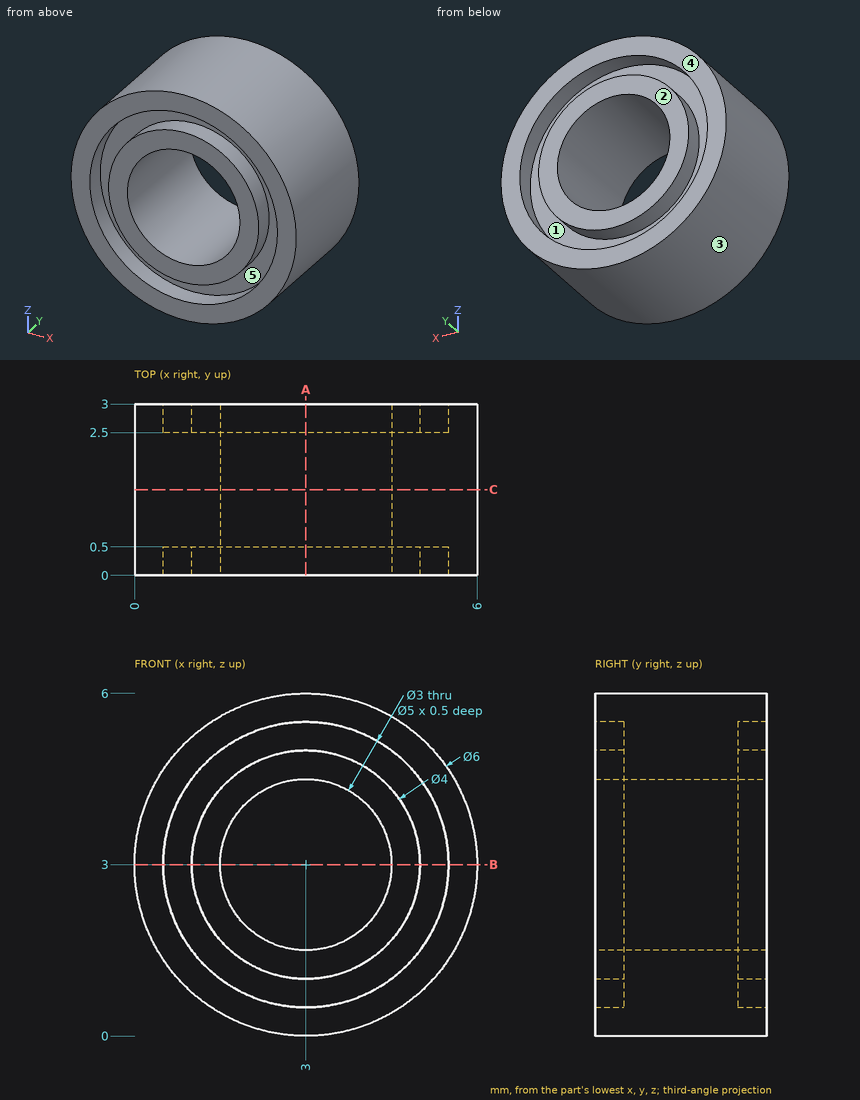
Geometry: see drawing. Coordinates: mm, zero at the bounding-box minimum. A direction names the side the tool comes from. Give positions to 0.01 mm unless a question says otherwise; leave off trailing zeros. Loops run counter-clockwise (first coordinate to the right, second up) from the corner with the lowest first, then second, coordinate; pieces in that order, holes last. Notation, with made-up numbers: (16.5, -34.75) -> (56.5, -34.75) arc R28 ccw to (56.5, -16.75) -> close; hole circle Ø8 at (10, 18.25). An arc over 180 degrees is marked (long way). Answer as a JSON object with one key per item and string values. Group by question number.
Item 1: Line query: probe 1 along X at (y, z) = (0.1, 3); probe 2 along Z at (x, y) = (1.45, 0.3); probe 3 along Z at (x, y) = (2.45, 0.2). Output: solid intervals per line, ascending.
Item 2: Pull-direction query (Z, two-part tool) for the marked faces 3, 4 and 5; classes: released by +Z, released by -Z, zero draft, split by the parting line, or undercut.
Item 3: Cut plane A-A, the plane x = 3. Return the cut outline in (y, z), and give its area (3 significant figures).
Item 4: Cut plane C-C, the plane y = 1.5. Return the cut outline in (x, z), and give its area (3 significant figures).
Item 5: Reachability of the marked faces 1 and 2 from +Z, -Z, +X, -X, +Y, -Y: full face, straight path, thin tool, end or side. Return the list, or none.
Item 6: Cut plane B-B, the plane z = 3. Return the cut outline in (x, y).
Item 7: Pin query (flat end, axial travel): P1, Ø1, axis at x = 4.5, y = 2, coming from the +Z side; P2, Ø1.5, axis at x = 2.5, y = 1, coming from the +Z side. Return the tip coordinate at first contact, or that it passes through.
Checks:
{
 "1": {"probe 1": "x = 0 to 0.5, 1 to 1.5, 4.5 to 5, 5.5 to 6", "probe 2": "z = 0.43 to 1.04, 1.74 to 4.26, 4.96 to 5.57", "probe 3": "z = 0.05 to 0.56, 1.08 to 1.6, 4.4 to 4.92, 5.44 to 5.95"},
 "2": {"face 3": "split by the parting line", "face 4": "zero draft", "face 5": "undercut"},
 "3": {"outline": "(0, 0) -> (3, 0) -> (3, 0.5) -> (2.5, 0.5) -> (2.5, 1) -> (3, 1) -> (3, 1.5) -> (0, 1.5) -> (0, 1) -> (0.5, 1) -> (0.5, 0.5) -> (0, 0.5) -> close; (0, 4.5) -> (3, 4.5) -> (3, 5) -> (2.5, 5) -> (2.5, 5.5) -> (3, 5.5) -> (3, 6) -> (0, 6) -> (0, 5.5) -> (0.5, 5.5) -> (0.5, 5) -> (0, 5) -> close", "area": "8.00 mm²"},
 "4": {"outline": "circle Ø6 at (3, 3); hole circle Ø3 at (3, 3)", "area": "21.2 mm²"},
 "5": {"face 1": "+Y", "face 2": "+Z, -Z, +X, -X, +Y"},
 "6": {"outline": "(0, 0) -> (0.5, 0) -> (0.5, 0.5) -> (1, 0.5) -> (1, 0) -> (1.5, 0) -> (1.5, 3) -> (1, 3) -> (1, 2.5) -> (0.5, 2.5) -> (0.5, 3) -> (0, 3) -> close; (4.5, 0) -> (5, 0) -> (5, 0.5) -> (5.5, 0.5) -> (5.5, 0) -> (6, 0) -> (6, 3) -> (5.5, 3) -> (5.5, 2.5) -> (5, 2.5) -> (5, 3) -> (4.5, 3) -> close"},
 "7": {"P1": "stops at z = 5.83", "P2": "stops at z = 6"}
}
